The model under review builds one solid part; all positions refer to its coordinate system, in mm. A direction names the side the tool comes from. Coordinates: 2 decimals unless noted, no trailing zeros. Order: outer loops, then holes, each group sorted by start corner. A loop starts at its lowest first (then second) coordinate and runs counter-clockwise, first axis right, second up.
```python
from build123d import *

# Parameters (mm, degrees)
SKETCH1_W           = 19.05
SKETCH1_H           = 50.8
BOSS_EXTRUDE1_DEPTH = 6.35
CUT_EXTRUDE1_START  = -7.35
SKETCH2_R           = 1.7272
CUT_EXTRUDE1_DEPTH  = 8.35
SKETCH3_R           = 2.54
CUT_EXTRUDE2_DEPTH  = 3.175
SKETCH4_W           = 4.8006
SKETCH4_H           = 13.97
CUT_EXTRUDE3_DEPTH  = 7.35
FILLET2_R           = 1.5


with BuildPart() as part:
    # Sketch1 → Boss-Extrude1 (new body)
    with BuildSketch(Plane(origin=(0, 0, 0), x_dir=(1, 0, 0), z_dir=(0, 1, 0))):
        Rectangle(SKETCH1_W, SKETCH1_H)
    extrude(amount=BOSS_EXTRUDE1_DEPTH)

    # Sketch2 → Cut-Extrude1 (cut)
    with BuildSketch(Plane(origin=(0, 6.35, 0), x_dir=(1, 0, 0), z_dir=(0, 1, 0)).offset(CUT_EXTRUDE1_START)):
        with Locations((0, 4.7625)):
            Circle(SKETCH2_R)
    cut_extrude1 = extrude(amount=CUT_EXTRUDE1_DEPTH, mode=Mode.SUBTRACT)

    # Sketch3 → Cut-Extrude2 (cut)
    with BuildSketch(Plane(origin=(0, 6.35, 0), x_dir=(1, 0, 0), z_dir=(0, 1, 0))):
        with Locations((0, 4.7625)):
            Circle(SKETCH3_R)
    cut_extrude2 = extrude(amount=-CUT_EXTRUDE2_DEPTH, mode=Mode.SUBTRACT)

    # Sketch4 → Cut-Extrude3 (cut, through all)
    with BuildSketch(Plane(origin=(0, 6.35, 0), x_dir=(1, 0, 0), z_dir=(0, 1, 0))):
        with Locations((0, 18.415)):
            Rectangle(SKETCH4_W, SKETCH4_H)
    cut_extrude3 = extrude(amount=-CUT_EXTRUDE3_DEPTH, mode=Mode.SUBTRACT)

    # Mirror1: Cut-Extrude1, Cut-Extrude2, Cut-Extrude3 across plane
    add(cut_extrude1.mirror(Plane.XY), mode=Mode.SUBTRACT)
    add(cut_extrude2.mirror(Plane.XY), mode=Mode.SUBTRACT)
    add(cut_extrude3.mirror(Plane.XY), mode=Mode.SUBTRACT)

    # Fillet2
    fillet2_edges = [part.edges().sort_by_distance(p)[0] for p in [
        (2.4003, 3.175, -11.43),
        (-2.4003, 3.175, -11.43),
        (2.4003, 3.175, 11.43),
        (-2.4003, 3.175, 11.43),
        (9.525, 3.175, 25.4),
        (-9.525, 3.175, 25.4),
        (-9.525, 3.175, -25.4),
        (9.525, 3.175, -25.4),
    ]]
    fillet(fillet2_edges, radius=FILLET2_R)


solid = part.part
```
(1) We need section B-B, the plane x = 0. Count the separate pieces of the cut face and the enclosed holes in it, and give its area (3 significant figures).
A:
separate pieces: 3
enclosed holes: 0
area: 91.0 mm2
(2) Wall thickness on probe 1 along Z at (x, y) = (0, 3.9); probe 2 along Z at (x, y) = (0, 1.05); probe 3 along X at (y, z) = (0.5, 21.5) (3 decimals): over which ranges is each line inside the solid? List them lowest first.
A:
probe 1: z = -11.43 to -7.3, -2.22 to 2.22, 7.3 to 11.43
probe 2: z = -11.43 to -6.49, -3.04 to 3.04, 6.49 to 11.43
probe 3: x = -9.525 to -2.4, 2.4 to 9.525
(3) We need section C-C, the plane y = 2. Write out the cut boundary in (x, z) (1 decimal).
A:
outline: (-9.5, -23.9) arc R1.5 ccw to (-8, -25.4) - (-2.4, -25.4) - (-2.4, -12.9) arc R1.5 cw to (-0.9, -11.4) - (0.9, -11.4) arc R1.5 cw to (2.4, -12.9) - (2.4, -25.4) - (8, -25.4) arc R1.5 ccw to (9.5, -23.9) - (9.5, 23.9) arc R1.5 ccw to (8, 25.4) - (2.4, 25.4) - (2.4, 12.9) arc R1.5 cw to (0.9, 11.4) - (-0.9, 11.4) arc R1.5 cw to (-2.4, 12.9) - (-2.4, 25.4) - (-8, 25.4) arc R1.5 ccw to (-9.5, 23.9) - close; hole circle Ø3.5 at (0, -4.8); hole circle Ø3.5 at (0, 4.8)
(4) For pin 1 Ø0.9 at (x, y) = (0.5, 3) entering from -Z; pin 2 Ø2 at (x, y) = (0.5, 4) entering from +Z; pin 3 Ø1.5 at (x, z) = (1.5, 15) entering from -Y; pin 4 Ø1.5 at (x, y) = (-0.5, 1.5) entering from -Z, all flat-tipped, find the tip position at first contact; note any pin that passes through.
A:
pin 1: stops at z = -11.43
pin 2: stops at z = 11.56
pin 3: passes through
pin 4: stops at z = -11.47
(5) We need section A-A, the plane z = -13.5. Write out the cut boundary in (x, y) (3 decimals).
A:
outline: (-9.525, 0) - (-2.4, 0) - (-2.4, 6.35) - (-9.525, 6.35) - close; (2.4, 0) - (9.525, 0) - (9.525, 6.35) - (2.4, 6.35) - close
(6) Machinability: for faces 5 (the face through (-0.225, 1.565, 6.475)), 6 (the face through (2.4, 3, -19)), 7 (the face through (2, 3.175, -4)), which of the approach directions +Z, -Z, +X, -X, +Y, -Y give a long, thin tool a straight path to every point of the face, cutting with its end or side? Answer none if there is none.
A:
face 5: +Y, -Y
face 6: -Z, +Y, -Y
face 7: +Y
(7) We need section D-D, the plane y = 5.5. Write out the cut boundary in (x, z) (1 decimal), and give its area (3 significant figures).
A:
outline: (-9.5, -23.9) arc R1.5 ccw to (-8, -25.4) - (-2.4, -25.4) - (-2.4, -12.9) arc R1.5 cw to (-0.9, -11.4) - (0.9, -11.4) arc R1.5 cw to (2.4, -12.9) - (2.4, -25.4) - (8, -25.4) arc R1.5 ccw to (9.5, -23.9) - (9.5, 23.9) arc R1.5 ccw to (8, 25.4) - (2.4, 25.4) - (2.4, 12.9) arc R1.5 cw to (0.9, 11.4) - (-0.9, 11.4) arc R1.5 cw to (-2.4, 12.9) - (-2.4, 25.4) - (-8, 25.4) arc R1.5 ccw to (-9.5, 23.9) - close; hole circle Ø5.1 at (0, -4.8); hole circle Ø5.1 at (0, 4.8)
area: 793 mm2
(8) Draft analysis for pull direction X (two halves, no side actions). For faces 1 (the face through (5, 3, -25.4)), 2 (the face through (9.525, 3, 0)), 3 (the face through (-1.97, 3.13, 11.88)), 4 (the face through (1.97, 3.13, 11.88)), state which applies: released by +X, released by -X, zero draft, split by the parting line, or undercut.
A:
face 1: zero draft
face 2: released by +X
face 3: undercut
face 4: undercut
